The figure shows three views and two pictorial views of one solid part (mm, origin at its lowest corner). Answer the questions. A direction names the side the tool comes from. Give positions to 0.01 mm unless a question says otherwise; leave off trailing zeros. Write each loop counter-clockwise with the first axis right and the second up, starting at its lowest first coordinate (ties: lowest second). Pieces come first, ordered by that corner, then holes. Notation, with made-up numbers: M -30,12.5 L 6,12.5 A31 ccw 6,39.5 Z; hole C 28,-14 d2. An arc over 180 degrees is marked long. Return JSON: item names as keys, results as strings.
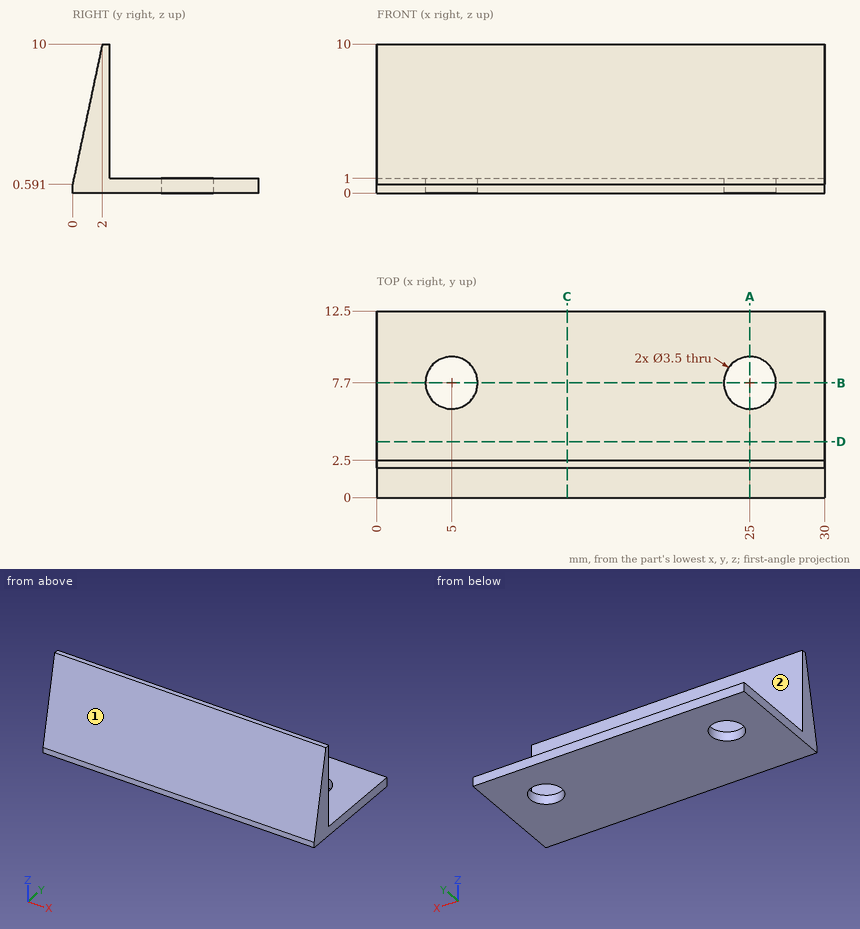
Item 1: A cutting plane is placed at C-C, the plane x = 12.75. Write down the section's boundary in (y, z).
Geometry results:
{"outline": "M 0,0 L 12.5,0 L 12.5,1 L 2.5,1 L 2.5,10 L 2,10 L 0,0.59 Z"}
Item 2: Given pin 1 Ø2 at (x, y) = (25, 7.7) entering from +Z; pin 2 Ø1.5 at (x, y) = (6.5, 4) entering from -Z; pin 3 Ø2.5 at (x, z) = (19.5, 4.5) entering from +Y; pin 4 Ø5 at (x, y) = (8.5, 6.5) entering from +Z, each flat-ended and moving along its own axis, determine where each tip first touches the part or whether it passes through.
Geometry results:
{"pin 1": "passes through", "pin 2": "stops at z = 0", "pin 3": "stops at y = 2.5", "pin 4": "stops at z = 1"}
Item 3: Find the intervals of material crossed by line 1 (Y direction, x = 5, z = 0.3); line 2 (Z direction, x = 28.25, y = 11); line 3 (Y direction, x = 23.75, z = 8) (1 decimal), in increasing order.
Geometry results:
{"line 1": "y = 0 to 5.95, 9.45 to 12.5", "line 2": "z = 0 to 1", "line 3": "y = 1.6 to 2.5"}
Item 4: A cutting plane is placed at B-B, the plane y = 7.7. Write down the section's boundary in (x, z).
Geometry results:
{"outline": "M 0,0 L 3.25,0 L 3.25,1 L 0,1 Z; M 6.75,0 L 23.25,0 L 23.25,1 L 6.75,1 Z; M 26.75,0 L 30,0 L 30,1 L 26.75,1 Z"}
Item 5: A cutting plane is placed at D-D, the plane y = 3.75. Write down the section's boundary in (x, z).
Geometry results:
{"outline": "M 0,0 L 30,0 L 30,1 L 0,1 Z"}
Item 6: A cutting plane is placed at A-A, the plane x = 25. Write down the section's boundary in (y, z), plus the area to 3 significant figures.
Geometry results:
{"outline": "M 0,0 L 5.95,0 L 5.95,1 L 2.5,1 L 2.5,10 L 2,10 L 0,0.59 Z; M 9.45,0 L 12.5,0 L 12.5,1 L 9.45,1 Z", "area": "22.1 mm2"}
Item 7: Which of the six approach directions +Z, -Z, +X, -X, +Y, -Y give full straight-line access (tool end or side, diameter ignored) to the marked faces 1 and 2?
Geometry results:
{"face 1": "+Z, +X, -X, -Y", "face 2": "+Z, +X, -X, +Y"}
